Read the model definition and answer for the solid it produces. Units are mm, in the model's axes. Face numbers are marked on the shaded views. A direction names the side the tool comes from. Coordinates: 2 decimals unless noted, no trailing zeros. Order: outer loops, then holes, each group sorted by start corner. A loop starts at its lowest first (then second) coordinate and runs counter-clockwise, first axis right, second up. Notation, with made-up numbers: (-5.5, 56.5) - (52.5, 56.5) arc R21 ccw to (52.5, 80.5) - close; hole circle Ø1 at (47.5, 26.25). An arc over 180 degrees is marked (long way). Write item = value, one per line.
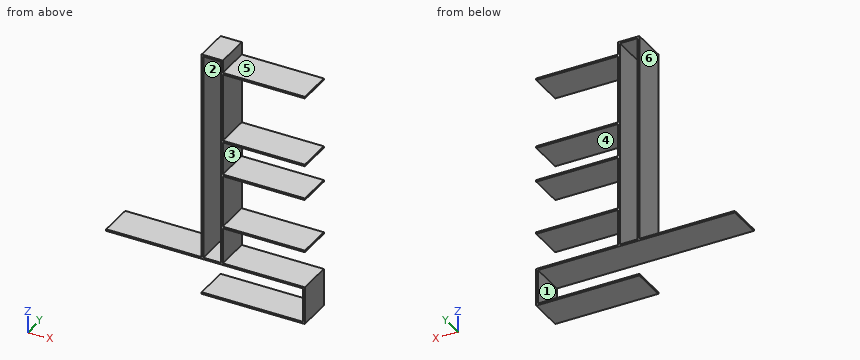
from build123d import *

# Parameters (mm, degrees)
SKETCH1_W           = 110.5
SKETCH1_H           = 2
SKETCH1_W_2         = 119.5
SKETCH1_W_3         = 2
SKETCH1_H_2         = 40
SKETCH1_W_4         = 20.5
SKETCH1_W_5         = 95
BOSS_EXTRUDE1_DEPTH = 40
SKETCH1_4_W         = 20.5
SKETCH1_4_H         = 2
BOSS_EXTRUDE2_DEPTH = 40


with BuildPart() as part:
    # Sketch1 → Boss-Extrude1 (new body)
    with BuildSketch(Plane(origin=(0, 0, 0), x_dir=(1, 0, 0), z_dir=(0, 1, 0))):
        with Locations((-79.75, 244)):
            Rectangle(SKETCH1_W, SKETCH1_H)
        with Locations((35.25, 286)):
            Rectangle(SKETCH1_W_2, SKETCH1_H)
        with Locations((94, 265)):
            Rectangle(SKETCH1_W_3, SKETCH1_H_2)
        Polygon((0, 245), (0, 243), (95, 243), (95, 245), (93, 245), align=None)
        with Locations((-12.25, 244)):
            Rectangle(SKETCH1_W_4, SKETCH1_H)
        with Locations((-1, 244)):
            Rectangle(SKETCH1_W_3, SKETCH1_H)
        Polygon((0, 0), (0, 14.7), (0, 16.7), (0, 96), (0, 98), (0, 136.5), (0, 138.5), (0, 199), (0, 201), (0, 243), (-2, 243), (-2, 2), (-2, 0), align=None)
        with Locations((-23.5, 244)):
            Rectangle(SKETCH1_W_3, SKETCH1_H)
        Polygon((-24.5, 0), (-22.5, 0), (-22.5, 2), (-22.5, 243), (-24.5, 243), align=None)
        with Locations((47.5, 137.5)):
            Rectangle(SKETCH1_W_5, SKETCH1_H)
        with Locations((47.5, 97)):
            Rectangle(SKETCH1_W_5, SKETCH1_H)
        with Locations((47.5, 15.7)):
            Rectangle(SKETCH1_W_5, SKETCH1_H)
        with Locations((47.5, 200)):
            Rectangle(SKETCH1_W_5, SKETCH1_H)
    extrude(amount=BOSS_EXTRUDE1_DEPTH)

    # Sketch1_4 → Boss-Extrude2 (add)
    with BuildSketch(Plane(origin=(0, 0, 0), x_dir=(1, 0, 0), z_dir=(0, 1, 0))):
        with Locations((-12.25, 1)):
            Rectangle(SKETCH1_4_W, SKETCH1_4_H)
    extrude(amount=BOSS_EXTRUDE2_DEPTH)


solid = part.part
1) The part is cut by section D-D (x = 74). Determine the outline of the cut face in (y, z), and give its area (3 significant figures).
Returned:
outline = (0, -287) - (40, -287) - (40, -285) - (0, -285) - close; (0, -245) - (40, -245) - (40, -243) - (0, -243) - close; (0, -201) - (40, -201) - (40, -199) - (0, -199) - close; (0, -138.5) - (40, -138.5) - (40, -136.5) - (0, -136.5) - close; (0, -98) - (40, -98) - (40, -96) - (0, -96) - close; (0, -16.7) - (40, -16.7) - (40, -14.7) - (0, -14.7) - close
area = 480 mm^2
2) The part is cut by section C-C (z = -87.5). Determine the outline of the cut face in (x, y).
Returned:
outline = (-24.5, 0) - (-22.5, 0) - (-22.5, 40) - (-24.5, 40) - close; (-2, 0) - (0, 0) - (0, 40) - (-2, 40) - close
3) The part is cut by section A-A (x = -11.5). Determine the outline of the cut face in (y, z).
Returned:
outline = (0, -287) - (40, -287) - (40, -285) - (0, -285) - close; (0, -245) - (40, -245) - (40, -243) - (0, -243) - close; (0, -2) - (40, -2) - (40, 0) - (0, 0) - close
4) Flat-ended cylindrical pins translate along their axes: pin 1 Ø12 at (y, z) = (7.5, -241.5) entering from -X; pin 2 Ø12 at (y, z) = (20, -66) entering from +X; pin 3 Ø12 at (x, y) = (46.5, 24.5) entering from +Z; pin 4 Ø3 at (x, y) = (-65, 16) entering from -Z. Find the tip coordinate at first contact, or state that the pin passes through.
Returned:
pin_1 = -135
pin_2 = 0
pin_3 = -14.7
pin_4 = -245
5) Determine the mould class of the marked faces 4, 5 and 6 for opening direction Z: pulls with the +Z half, pulls with the -Z half, needs draft (parallel to the pull), parting line crosses it, or undercut.
Returned:
face_4 = undercut
face_5 = pulls with the +Z half
face_6 = needs draft
6) For the marked faces 1, 2 and 3, determine the directions among +Z, -Z, +X, -X, +Y, -Y from which every point of the face is accessible in a straight line to the end or side of a thin tool.
Returned:
face_1 = -X, +Y, -Y
face_2 = +Y, -Y
face_3 = +X, +Y, -Y
7) Straight lines are drawn through the part: line 1 along Z through (x, y) = (8.5, 7); line 2 along X through (y, z) = (29, -110); line 3 along X through (y, z) = (34, -137.5). For each, find the intervals that lie inside material, in ascending order. Write a range as from..to.
Returned:
line_1 = -287..-285, -245..-243, -201..-199, -138.5..-136.5, -98..-96, -16.7..-14.7
line_2 = -24.5..-22.5, -2..0
line_3 = -24.5..-22.5, -2..95
